Build history of the part. All positions in model axes, mm. Face numbers are marked on the shaded views. A direction names the side the tool comes from. Give positions to 0.01 mm unless a question says otherwise; leave off trailing zeros. Loops run counter-clockwise (first coordinate to the right, second up) from the corner with the lowest first, then second, coordinate; pieces in that order, holes last. Notation, with made-up numbers: (42.5, 0.25) -> (81.5, 0.25) arc R32 ccw to (81.5, 39.25) -> close; hole circle Ø8 at (-4, -13.75). An arc over 180 degrees is marked (long way). One line per question, with ' | ' between items. Start each with the question number.
(1) Flat gauge pins, fed straight in: pin 1 Ø1.5 at (y, z) = (6.5, 0.5) entering from +X; pin 2 Ø2 at (x, y) = (1.5, 5.5) entering from -Z; pin 3 Ø1 at (y, z) = (4.5, 0) entering from -X. Where does each tip first touch, or does it go through?
(2) Slice it at C-C, the plane x = 0.55. Write the cut outline in (y, z).
(3) Slice it at A-A, the plane y = 4.25. Write the cut outline in (x, z).
(4) 3-axis set-ups, long thin cutter, end or side, ignore diameter. For the marked faces 1 and 2: which of +Z, -Z, +X, -X, +Y, -Y reach the whole face in a straight line?
(5) Drill centre lines: L1, parallel to Y at x = -0.45, z = 1.15; L2, parallel to Z at x = 0.25, y = 7.75; L3, parallel to X at y = 6.7, z = 0. Where is each one in solid material? Low to high. Write a range as from..to.
(6) Slice it at B-B, the plane z = -0.35. Write the cut outline in (x, y).
(7) Slice it at D-D, the plane y = 1.75. Write the cut outline in (x, z).
(8) Mould opens along Z. For the marked faces 3, 4, 5 and 6 say: pulls with the +Z half, pulls with the -Z half, needs draft (parallel to the pull), parting line crosses it, or undercut.
```python
from build123d import *

# Parameters (mm, degrees)
SKETCH1_R           = 1
BOSS_EXTRUDE1_DEPTH = 3
BOSS_EXTRUDE2_DEPTH = 6
CUT_EXTRUDE1_START  = -5
SKETCH3_R           = 1
CUT_EXTRUDE1_DEPTH  = 5


with BuildPart() as part:
    # Sketch1 → Boss-Extrude1 (new body)
    with BuildSketch(Plane(origin=(0, 0, 0), x_dir=(1, 0, 0), z_dir=(0, 1, 0))):
        with Locations(Location((0, 0, 0), (0, 0, 270))):
            Circle(SKETCH1_R)
    extrude(amount=BOSS_EXTRUDE1_DEPTH)

    # Sketch2 → Boss-Extrude2 (add)
    with BuildSketch(Plane(origin=(0, 3, 0), x_dir=(1, 0, 0), z_dir=(0, 1, 0))):
        Polygon((-0.306435831, -2.289584478), (1.829620407, -1.410173453), (2.136056237, 0.879411025), (0.306435831, 2.289584478), (-1.829620407, 1.410173453), (-2.136056237, -0.879411025), align=None)
    extrude(amount=BOSS_EXTRUDE2_DEPTH)

    # Sketch3 → Cut-Extrude1 (cut)
    with BuildSketch(Plane(origin=(0, 9, 0), x_dir=(1, 0, 0), z_dir=(0, 1, 0)).offset(CUT_EXTRUDE1_START)):
        with Locations(Location((0, 0, 0), (0, 0, 270))):
            Circle(SKETCH3_R)
    extrude(amount=CUT_EXTRUDE1_DEPTH, mode=Mode.SUBTRACT)


solid = part.part
```
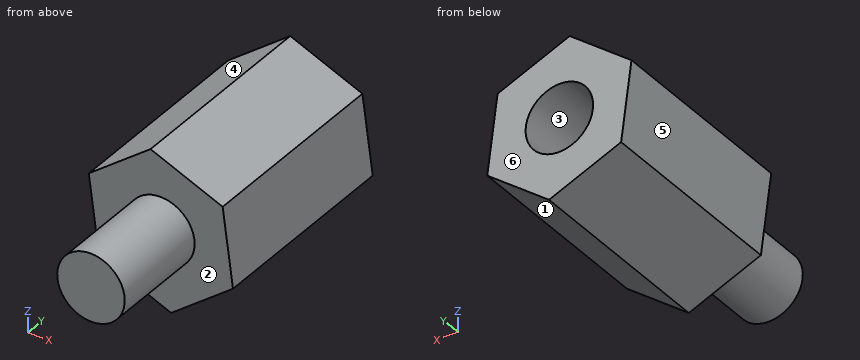
Final values:
1) pin 1: x = 2.05 | pin 2: z = -2.14 | pin 3: x = -2.09
2) outline: (0, -0.84) -> (3, -0.84) -> (3, -2.1) -> (9, -2.1) -> (9, -0.84) -> (4, -0.84) -> (4, 0.84) -> (9, 0.84) -> (9, 1.94) -> (3, 1.94) -> (3, 0.84) -> (0, 0.84) -> close
3) outline: (-2.14, 0.88) -> (-1.83, -1.41) -> (0.31, -2.29) -> (2.14, -0.88) -> (1.83, 1.41) -> (-0.31, 2.29) -> close; hole circle Ø2 at (0, 0)
4) face 1: -Z, +X, +Y, -Y | face 2: -Y
5) L1: 3..9 | L2: -2.27..-0.97, 0.97..2.06 | L3: -2.02..-1, 1..2.02
6) outline: (-1.97, 3) -> (-0.94, 3) -> (-0.94, 0) -> (0.94, 0) -> (0.94, 3) -> (2.07, 3) -> (2.07, 9) -> (0.94, 9) -> (0.94, 4) -> (-0.94, 4) -> (-0.94, 9) -> (-1.97, 9) -> close
7) outline: circle Ø2 at (0, 0)
8) face 3: undercut | face 4: pulls with the +Z half | face 5: pulls with the -Z half | face 6: needs draft
